For this review, use the dimensioned drawing (mm, ordinates from the lowest corner) and the shaded views. A direction names the side the tool comes from. Coordinates: 2 decimals unless noted, no trailing zeros. Write each loop counter-clockwise with the first axis right and the second up, starting at its lowest first coordinate (ties: lowest second). Pieces come first, ordered by that corner, then holes.
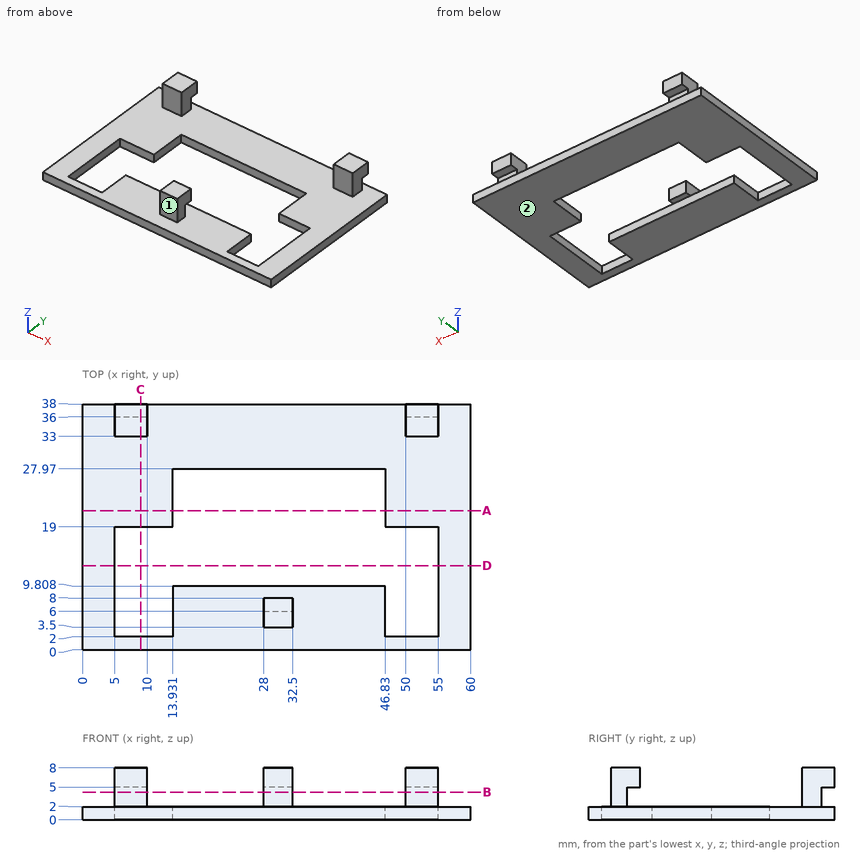
(1) For the marked faces 1 and 2, list the 3-axis set-ups (+Z, -Z, +X, -X, +Y, -Y) from which the entire face can be reached by the end or side of a thin tool; tool diameter is ignored.
(2) Consider section A-A (y = 21.5). Give the boundary of the cut face in (x, z).
(3) Insertion check: pin 1 Ø4 at (y, z) = (35.5, 4.5) entering from -X; pin 2 Ø12 at (x, y) = (19, 26.5) entering from +Z; pin 3 Ø4 at (x, z) = (53.5, 4.5) entering from -Y; pin 4 Ø11.5 at (x, y) = (39.5, 18) entering from +Z. Each pin has a flat end and moves straight along its axis. Give the tip position at first contact, or say it passes through.
(4) Wall thickness on line 1 (X direction, y = 18, z = 1.25); line 2 (X direction, y = 36, z = 6.75); line 3 (Y direction, x = 43.5, z = 0.75): over which ranges is each line inside the solid? List them lowest first.
(5) Consider section B-B (z = 4.25). Give the boundary of the cut face in (x, y).
(6) Consider section C-C (x = 9). Give the boundary of the cut face in (y, z).
(7) Consider section D-D (y = 13). Give the boundary of the cut face in (x, z).
Results:
1. face 1: +Z, +X, -X, -Y
1. face 2: -Z, +X, -X, +Y, -Y
2. outline: (0, 0) - (13.93, 0) - (13.93, 2) - (0, 2) - close; (46.83, 0) - (60, 0) - (60, 2) - (46.83, 2) - close
3. pin 1: stops at x = 5
3. pin 2: stops at z = 2
3. pin 3: stops at y = 33
3. pin 4: passes through
4. line 1: x = 0 to 5, 55 to 60
4. line 2: x = 5 to 10, 50 to 55
4. line 3: y = 0 to 9.81, 27.97 to 38
5. outline: (5, 33) - (10, 33) - (10, 36) - (5, 36) - close; (28, 3.5) - (32.5, 3.5) - (32.5, 6) - (28, 6) - close; (50, 33) - (55, 33) - (55, 36) - (50, 36) - close
6. outline: (0, 0) - (2, 0) - (2, 2) - (0, 2) - close; (19, 0) - (38, 0) - (38, 2) - (36, 2) - (36, 5) - (38, 5) - (38, 8) - (33, 8) - (33, 2) - (19, 2) - close
7. outline: (0, 0) - (5, 0) - (5, 2) - (0, 2) - close; (55, 0) - (60, 0) - (60, 2) - (55, 2) - close
